Work out the finished part from the listing and answer in its coordinate system (mm). Face numbers are marked on the shaded views. Round coordinates to 2 decimals unless told otherwise and drop trailing zeros. Order: outer loops, then holes, each group sorted by start corner. A loop starts at its lowest first (then second) coordinate and runs counter-clockwise, first axis right, second up. Notation, with made-up numbers: M -8.75,57 L 13.25,57 A16 cw 13.25,75 Z; hole C 35.25,9.25 d3. An arc over 180 degrees is marked long. Return JSON: item names as keys, results as strings.
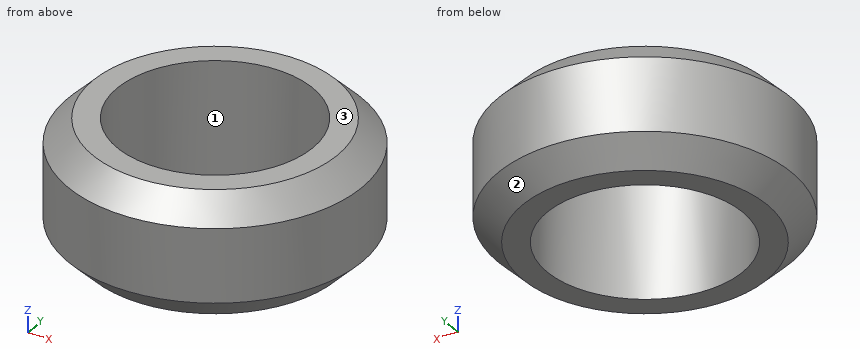
from build123d import *

# Parameters (mm, degrees)
CYLINDER017_R     = 8
CYLINDER017_DEPTH = 10
CYLINDER016_R     = 12
CYLINDER016_DEPTH = 10
CHAMFER008_SIZE   = 2


with BuildPart() as cylindre001:
    # Cylinder017 → Cylinder017 (new body)
    with BuildSketch(Plane.XY):
        Circle(CYLINDER017_R)
    extrude(amount=CYLINDER017_DEPTH)


with BuildPart() as chamfer008:
    # Cylinder016 → Cylinder016 (new body)
    with BuildSketch(Plane.XY):
        Circle(CYLINDER016_R)
    extrude(amount=CYLINDER016_DEPTH)

    # Cut008: cut Cylindre001
    add(cylindre001.part, mode=Mode.SUBTRACT)

    # Chamfer008
    chamfer008_edges = [chamfer008.edges().sort_by_distance(p)[0] for p in [
        (-12, 0, 10),
        (-12, 0, 0),
    ]]
    chamfer(chamfer008_edges, length=CHAMFER008_SIZE)


solid = chamfer008.part
Item 1: Find section C-C (z = 3.75). Determine the outline of the cut face in (x, y).
Output:
{"outline": "C 0,0 d24; hole C 0,0 d16"}
Item 2: Consider line 1 along Y through (x, z) = (0, 2.5); line 2 along Y through (x, z) = (-3.25, 0.5); line 3 along X through (y, z) = (5, 8.25) (3 decimals). Determine where each line is inside the solid, lowest interval first. Write a range as [from, to].
Output:
{"line 1": "y = [-12, -8], [8, 12]", "line 2": "y = [-9.98, -7.31], [7.31, 9.98]", "line 3": "x = [-10.633, -6.245], [6.245, 10.633]"}
Item 3: Each of these flat-tipped pins is pushed along its axis until it touches: pin 1 (8 mm diameter, centred on x = -1.5, y = 9.5, fed in from -Z); pin 2 (3 mm diameter, centred on x = -2, z = 1, fed in from +Y); pin 3 (5 mm diameter, centred on y = -4, z = 6.5, fed in from +X); pin 4 (4 mm diameter, centred on x = 5.5, z = 6.5, fed in from -Y). Where does it stop, or does it pass through?
Output:
{"pin 1": "stops at z = 0", "pin 2": "stops at y = 11.97", "pin 3": "stops at x = 11.91", "pin 4": "stops at y = -11.48"}
Item 4: The mould has two halves that part along X. Classify the marked faces 1, 2 and 3: pulls with the +X half, pulls with the -X half, needs draft (parallel to the pull), parting line crosses it, or undercut.
Output:
{"face 1": "undercut", "face 2": "parting line crosses it", "face 3": "needs draft"}
Item 5: Find section A-A (x = 0). Determine the outline of the cut face in (y, z), plus the area to 3 significant figures.
Output:
{"outline": "M -12,2 L -10,0 L -8,0 L -8,10 L -10,10 L -12,8 Z; M 8,0 L 10,0 L 12,2 L 12,8 L 10,10 L 8,10 Z", "area": "72.0 mm^2"}
